Design review of the part built by this model. Coordinates are the model's own, in mm. A direction names the side the tool comes from. Coordinates: 2 decimals unless noted, no trailing zeros. Order: outer loops, then holes, each group sorted by start corner. A loop starts at its lowest first (then second) coordinate and runs counter-clockwise, first axis right, second up. Notation, with made-up numbers: M 70.5,60 L 120.5,60 A19 ccw 120.5,76 Z; hole C 2.25,30.25 d10. An arc over 180 degrees is marked long. Use CSV: the item, a comma, the result in double quotes.
```python
from build123d import *

# Parameters (mm, degrees)
SKETCH_R        = 17.5
PAD_DEPTH       = 15
SKETCH001_R     = 3.25
POCKET_DEPTH    = 15.001
POCKET001_DEPTH = 6
CHAMFER_SIZE    = 2


with BuildPart() as part:
    # Sketch → Pad (new body)
    with BuildSketch(Plane.XY):
        Circle(SKETCH_R)
    extrude(amount=PAD_DEPTH)

    # Sketch001 (on Face3 of Pad) → Pocket (cut, through all)
    with BuildSketch(Plane.XY.offset(15)):
        Circle(SKETCH001_R)
    extrude(amount=-POCKET_DEPTH, mode=Mode.SUBTRACT)

    # Sketch002 (on Face3 of Pocket) → Pocket001 (cut)
    with BuildSketch(Plane.XY.offset(15)):
        Polygon((2.886751, 5), (-2.886751, 5), (-5.773503, 0), (-2.886751, -5), (2.886751, -5), (5.773503, 0), align=None)
    extrude(amount=-POCKET001_DEPTH, mode=Mode.SUBTRACT)

    # Chamfer
    chamfer_edges = [part.edges().sort_by_distance(p)[0] for p in [
        (-17.5, 0, 15),
    ]]
    chamfer(chamfer_edges, length=CHAMFER_SIZE)


solid = part.part
```
(1) The part is to be moulded in two halves that separate along Y. For faces 3 (the face through (-0.1, 3.4, 9)), 4 (the face through (-13.887, -10.648, 6.409)), 5 (the face through (-4, 4, 15)), say which applies: pulls with the +Y half, pulls with the -Y half, needs draft (parallel to the pull), parting line crosses it, or undercut.
The answers:
face 3,"undercut"
face 4,"parting line crosses it"
face 5,"needs draft"
(2) Add section A-A on z = 9.5. State the section outline as (x, y) points, and give its area (3 significant figures).
The answers:
outline,"C 0,0 d35; hole M -5.77,0 L -2.89,-5 L 2.89,-5 L 5.77,0 L 2.89,5 L -2.89,5 Z"
area,"876 mm2"
(3) Add section D-D on z = 1.5. State the section outline as (x, y) points.
The answers:
outline,"C 0,0 d35; hole C 0,0 d6.5"
(4) Wall thickness on probe 1 along Y at (x, z) = (0, 4.75); probe 2 along X at (y, z) = (-1.5, 1.75); probe 3 along X at (y, z) = (-1, 14.75): over which ranges is each line inside the solid? List them lowest first.
The answers:
probe 1,"y = -17.5 to -3.25, 3.25 to 17.5"
probe 2,"x = -17.44 to -2.88, 2.88 to 17.44"
probe 3,"x = -15.72 to -5.2, 5.2 to 15.72"
(5) Add section C-C on z = 13.75. State the section outline as (x, y) points, and give its area (3 significant figures).
The answers:
outline,"C 0,0 d33.5; hole M -5.77,0 L -2.89,-5 L 2.89,-5 L 5.77,0 L 2.89,5 L -2.89,5 Z"
area,"795 mm2"
(6) Clearance check with flat-ended pins moving along their axes: P1, Ø8, axis at y = 4.5, z = 9, coming from the -X side; P2, Ø2, axis at y = 13, z = 12.5, coming from the -X side; P3, Ø6, axis at y = -12.5, z = 9, coming from the -X side; P4, Ø4, axis at x = 0, y = 0, coming from the +Z side. State where each tip first meets the part, or that it passes through.
The answers:
P1,"stops at x = -17.49"
P2,"stops at x = -12.74"
P3,"stops at x = -14.7"
P4,"passes through"
(7) Add section B-B on x = 0. State the section outline as (y, z) points.
The answers:
outline,"M -17.5,0 L -3.25,0 L -3.25,9 L -5,9 L -5,15 L -15.5,15 L -17.5,13 Z; M 3.25,0 L 17.5,0 L 17.5,13 L 15.5,15 L 5,15 L 5,9 L 3.25,9 Z"
(8) For faces 1 (the face through (0, -4, 0)), 2 (the face through (4.31, -2.535, 12.042)), list the 3-axis set-ups (+Z, -Z, +X, -X, +Y, -Y) from which the entire face can be reached by the end or side of a thin tool; tool diameter is ignored.
The answers:
face 1,"-Z, +X, -X, +Y, -Y"
face 2,"+Z"
